from build123d import *

# Parameters (mm, degrees)
SKETCH1_W           = 24
SKETCH1_H           = 3.375672593
SKETCH1_R           = 1.5
BOSS_EXTRUDE1_DEPTH = 3
SKETCH2_W           = 24
SKETCH2_H           = 3
BOSS_EXTRUDE2_DEPTH = 25
FILLET1_R           = 10
SKETCH3_R           = 1.5
CUT_EXTRUDE1_DEPTH  = 32.123129679


with BuildPart() as part:
    # Sketch1 → Boss-Extrude1 (new body)
    # profile 1 of 2: a face of its own
    with BuildSketch(Plane(origin=(0, 0, 0), x_dir=(1, 0, 0), z_dir=(0, 1, 0))):
        with Locations((0, 4.687836297)):
            Rectangle(SKETCH1_W, SKETCH1_H)
    # profile 2 of 2: a face of its own
    with BuildSketch(Plane(origin=(0, 0, 0), x_dir=(1, 0, 0), z_dir=(0, 1, 0))):
        with BuildLine():
            ThreePointArc((-10.5, -3), (-11.560660172, -2.560660172), (-12, -1.5))
            Line((-12, -1.5), (-12, 3))
            Line((-12, 3), (12, 3))
            Line((12, 3), (12, -1.5))
            ThreePointArc((12, -1.5), (11.560660172, -2.560660172), (10.5, -3))
            Line((10.5, -3), (-10.5, -3))
        make_face()
        with Locations(Location((10, 0, 0), (0, 0, 270))):
            Circle(SKETCH1_R, mode=Mode.SUBTRACT)
        with Locations(Location((-10, 0, 0), (0, 0, 270))):
            Circle(SKETCH1_R, mode=Mode.SUBTRACT)
    extrude(amount=BOSS_EXTRUDE1_DEPTH)

    # Sketch2 → Boss-Extrude2 (add)
    with BuildSketch(Plane(origin=(0, 3, 0), x_dir=(1, 0, 0), z_dir=(0, 1, 0))):
        with Locations((0, 4.875672593)):
            Rectangle(SKETCH2_W, SKETCH2_H)
    extrude(amount=BOSS_EXTRUDE2_DEPTH)

    # Fillet1
    fillet1_edges = [part.edges().sort_by_distance(p)[0] for p in [
        (12, 28, -4.875672593),
        (-12, 28, -4.875672593),
    ]]
    fillet(fillet1_edges, radius=FILLET1_R)

    # Sketch3 → Cut-Extrude1 (cut, through all)
    with BuildSketch(Plane.XY.offset(-3.375672593)):
        with Locations((0, 17)):
            Circle(SKETCH3_R)
    extrude(amount=-CUT_EXTRUDE1_DEPTH, mode=Mode.SUBTRACT)


solid = part.part
Geometry check sheet. Reference: the model listing, model coordinates, mm. A direction names the side the tool comes from. Coordinates: 2 decimals unless noted, no trailing zeros. Loops run counter-clockwise (first coordinate to the right, second up) from the corner with the lowest first, then second, coordinate; pieces in that order, holes last. Notation, with made-up numbers: (-36.5, -6.5) - (2.5, -6.5) arc R19 cw to (2.5, 21.5) - close; hole circle Ø4 at (60.25, -23). An arc over 180 degrees is marked (long way). Use one line per item in the form item = value. Start each with the question number.
Item 1: Gauge pin test, flat ends, axial feed: pin 1 (1.5 mm diameter, centred on x = -6, z = -0.5, fed in from +Y); pin 2 (5 mm diameter, centred on x = 2.5, y = 17, fed in from +Z). Record the tip position at first contact, or that the pin passes through.
Item 2: Mould release check, pull along X, two halves, no side actions. Record for faces 3 (the face through (0, 28, -5)), 4 (the face through (-0.195, 18.487, -4.855)), 5 (the face through (-11.55, 1.48, 2.57)): +X half, -X half, draft (parallel to the pull), parting line (faces both ways), or undercut.
Item 3: Thickness scan on probe 1 along X at (y, z) = (1.6, 0); probe 2 along Y at (x, z) = (0, -4.75); probe 3 along Z at (x, y) = (9.5, 7). Record the ranges inside material, lowest first.
Item 4: Section check C-C, the plane x = 0. Enter the section's corners in (y, z).
Item 5: Section check D-D, the plane z = -4. Enter the section's corners in (x, y), and give its area (3 significant figures).
Item 6: Section check A-A, the plane y = 17. Enter the section's corners in (x, z).
Item 7: Tool access check on faces 1 (the face through (12, 7, -4)), 2 (the face through (0, 3, 0)). Record the directions out of +Z, -Z, +X, -X, +Y, -Y that give a thin tool (end or side, any length) a straight path to the whole face; none if there is none.
Item 8: Section check B-B, the plane z = 0. Enter the section's corners in (x, y), and give its area (3 significant figures).
Computed:
q1.pin_1 = 3
q1.pin_2 = -3.38
q2.face_3 = draft
q2.face_4 = undercut
q2.face_5 = -X half
q3.probe_1 = -12 to -11.5, -8.5 to 8.5, 11.5 to 12
q3.probe_2 = 0 to 15.5, 18.5 to 28
q3.probe_3 = -6.38 to -3.38
q4.outline = (0, -6.38) - (15.5, -6.38) - (15.5, -3.38) - (3, -3.38) - (3, 3) - (0, 3) - close; (18.5, -6.38) - (28, -6.38) - (28, -3.38) - (18.5, -3.38) - close
q5.outline = (-12, 0) - (12, 0) - (12, 18) arc R10 ccw to (2, 28) - (-2, 28) arc R10 ccw to (-12, 18) - close; hole circle Ø3 at (0, 17)
q5.area = 622 mm2
q6.outline = (-12, -6.38) - (-1.5, -6.38) - (-1.5, -3.38) - (-12, -3.38) - close; (1.5, -6.38) - (12, -6.38) - (12, -3.38) - (1.5, -3.38) - close
q7.face_1 = +Z, -Z, +X, +Y, -Y
q7.face_2 = +Z, +X, -X, +Y
q8.outline = (-12, 0) - (-11.5, 0) - (-11.5, 3) - (-12, 3) - close; (-8.5, 0) - (8.5, 0) - (8.5, 3) - (-8.5, 3) - close; (11.5, 0) - (12, 0) - (12, 3) - (11.5, 3) - close
q8.area = 54.0 mm2
